from build123d import *

# Parameters (mm, degrees)
F0_R     = 1
F1_DEPTH = 4
F2_W     = 12
F2_H     = 2
F3_DEPTH = 8.249357


with BuildPart() as f1:
    # F0 (on Front) → F1 (new body)
    with BuildSketch(Plane.XZ):
        with BuildLine():
            Line((15, 8), (0, 8))
            ThreePointArc((0, 8), (-4, 4), (0, 0))
            Line((0, 0), (15, 1))
            Line((15, 1), (15, 8))
        make_face()
        with Locations((0, 4)):
            Circle(F0_R, mode=Mode.SUBTRACT)
    extrude(amount=F1_DEPTH)

    # F2 (on face) → F3 (cut, through all)
    with BuildSketch(Plane(origin=(0, 0, 0), x_dir=(0.997785, 0, 0.066519), z_dir=(0.066519, 0, -0.997785))):
        with Locations((0, 2)):
            Rectangle(F2_W, F2_H)
    extrude(amount=-F3_DEPTH, mode=Mode.SUBTRACT)


solid = f1.part
Source: CAD feature listing. Evaluate the final solid. Frame: model axes, mm. Coordinates: 2 decimals unless noted, no trailing zeros. Order: outer loops, then holes, each group sorted by start corner. A loop starts at its lowest first (then second) coordinate and runs counter-clockwise, first axis right, second up. Notation, with made-up numbers: M -5,-24.75 L 40,-24.75 A18 ccw 40,4.25 Z; hole C 51,-32.75 d3. An arc over 180 degrees is marked long. Write each question's results on one line, items separated by ' | '. Start each with the question number.
Item 1: Cut plane D-D (z = 1.5). Return loops of the section in (x, y).
Item 2: First-contact query: pin 1 Ø4 at (x, z) = (1, 5) entering from +Y. Flat tip, straight axial feed; report the tip coordinate or a pass-through.
Item 3: Cut plane B-B (z = 4). Return loops of the section in (x, y).
Item 4: Line query: probe 1 along X at (y, z) = (-3.3, 4); probe 2 along Y at (x, z) = (-2, 6.5); probe 3 along Z at (x, y) = (0, -0.4). Output: solid intervals per line, ascending.
Item 5: Cut plane A-A (y = -0.65). Return loops of the section in (x, z).
Item 6: Draft query along X for faces 1 (the face through (5, -4, 4)), 2 (the face through (5.737, -1.986, 4.146)), 3 (the face through (-0.13, -0.49, 4.99)). Return one class per face: pulls with the +X half, pulls with the -X half, needs draft (parallel to the pull), parting line crosses it, or undercut.
Item 7: Cut plane C-C (x = 3.25). Return loops of the section in (y, z), and give its area (3 significant figures).
Checked values:
1) outline: M -3.12,-4 L 15,-4 L 15,0 L -3.12,0 L -3.12,-1 L 5.91,-1 L 5.91,-3 L -3.12,-3 Z
2) pin 1: stops at y = 0
3) outline: M -4,-4 L -1,-4 L -1,-3 L -4,-3 Z; M -4,-1 L -1,-1 L -1,0 L -4,0 Z; M 1,-4 L 15,-4 L 15,0 L 1,0 L 1,-1 L 5.75,-1 L 5.75,-3 L 1,-3 Z
4) probe 1: x = -4 to -1, 1 to 15 | probe 2: y = -4 to -3, -1 to 0 | probe 3: z = 0 to 3, 5 to 8
5) outline: M 0,0 L 15,1 L 15,8 L 0,8 A4 ccw Z; hole C 0,4 d2
6) face 1: needs draft | face 2: pulls with the -X half | face 3: undercut
7) outline: M -4,0.22 L -3,0.22 L -3,8 L -4,8 Z; M -1,0.22 L 0,0.22 L 0,8 L -1,8 Z | area: 15.6 mm2
